The drawing under review shows one solid part. Ordinate dimensions are in mm from its lowest x, y, z. A direction names the side the tool comes from. Round coordinates to 2 decimals unless told otherwise and drop trailing zeros. Write each loop counter-clockwise with the first axis right and the second up, starting at its lowest first coordinate (ties: lowest second). Pieces come first, ordered by that corner, then holes. Notation, with made-up numbers: (58, 10) -> (95, 10) arc R17 cw to (95, 39) -> close; hole circle Ø11 at (84, 20.25). An arc over 180 degrees is marked (long way). Write item = value, one per line. Start each with the question number.
Item 1: Mouldability with a two-part tool opening along Z and no side actions: class the marked faces 4, 5, 6 and 7 as released by +Z, released by -Z, zero draft, split by the parting line, or undercut.
Item 2: Add section B-B, the plane z = 27.5. State the section outline as (x, y) points (1 decimal), then the cut area to 3 significant figures.
Item 3: Add section D-D, the plane z = 47. State the section outline as (x, y) points (1 decimal).
Item 4: Add section C-C, the plane y = 28. State the section outline as (x, z) points.
Item 5: Machinability: for the marked faces 1, 2 and 3, which of the approach directions +Z, -Z, +X, -X, +Y, -Y give a long, thin tool a straight path to every point of the face, cutting with its end or side? Answer none if there is none.
Item 6: To check wall thickness, follow L1, parallel to Y at x = 24.5, z = 45.5; L2, parallel to X at y = 8, z = 27 (1 decimal); L3, parallel to Z at x = 85, y = 6.75. State the ranges of each line that lie inside material, in increasing order.
Item 7: Add section A-A, the plane x = 17.5. State the section outline as (y, z) points.
Item 8: For pin 1 Ø2.5 at (y, z) = (1.5, 16) entering from -X (3 decimals); pin 2 Ø9 at (x, y) = (21.5, 40) entering from -Z; pin 3 Ø6 at (x, z) = (37.5, 41) entering from -Y, all flat-tipped, find the tip position at first contact; note any pin that passes through.
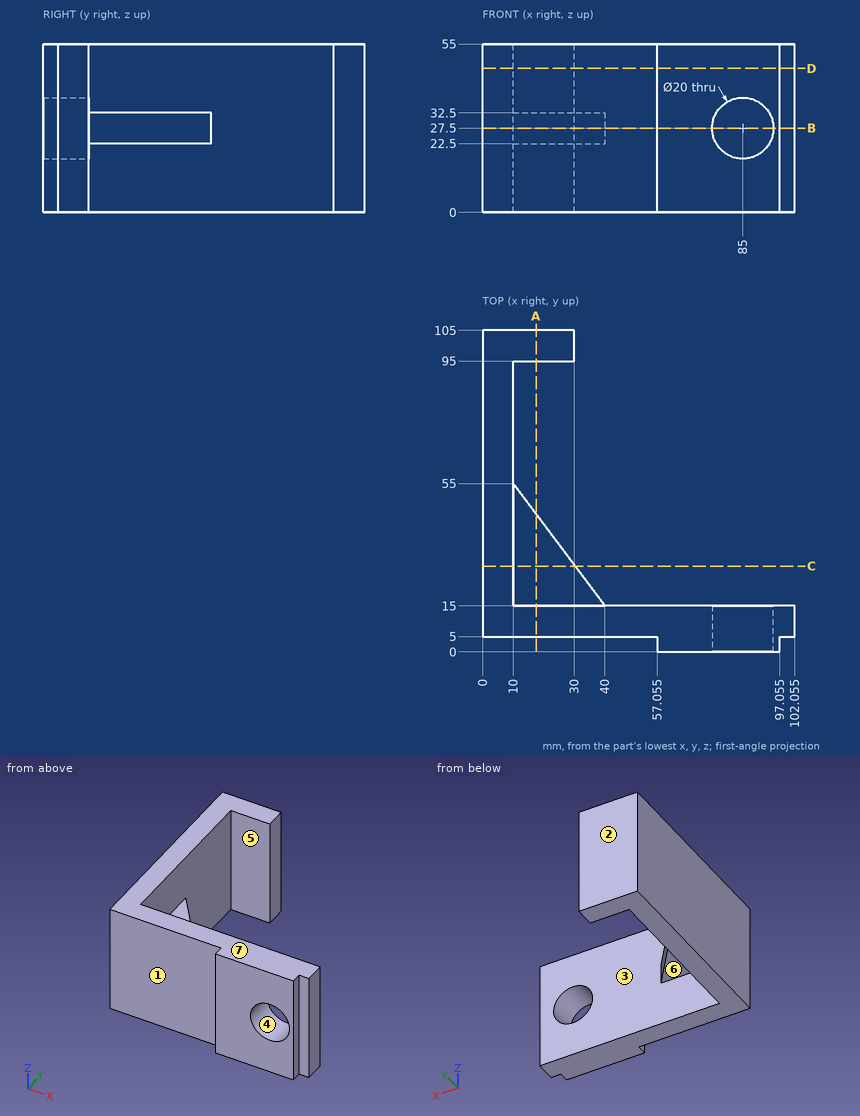
Result set:
q1.face_4 = undercut
q1.face_5 = zero draft
q1.face_6 = released by -Z
q1.face_7 = released by +Z
q2.outline = (0, 5) -> (57.1, 5) -> (57.1, 0) -> (75, 0) -> (75, 15) -> (40, 15) -> (10, 55) -> (10, 95) -> (30, 95) -> (30, 105) -> (0, 105) -> close; (95, 0) -> (97.1, 0) -> (97.1, 5) -> (102.1, 5) -> (102.1, 15) -> (95, 15) -> close
q2.area = 2,620 mm²
q3.outline = (0, 5) -> (57.1, 5) -> (57.1, 0) -> (97.1, 0) -> (97.1, 5) -> (102.1, 5) -> (102.1, 15) -> (10, 15) -> (10, 95) -> (30, 95) -> (30, 105) -> (0, 105) -> close
q4.outline = (0, 0) -> (10, 0) -> (10, 22.5) -> (30.25, 22.5) -> (30.25, 32.5) -> (10, 32.5) -> (10, 55) -> (0, 55) -> close
q5.face_1 = +Z, -Z, -X, -Y
q5.face_2 = +Z, -Z, +X, -X, +Y
q5.face_3 = +X
q6.L1 = 5 to 15, 95 to 105
q6.L2 = 0 to 75, 95 to 102.1
q6.L3 = 0 to 17.5, 37.5 to 55
q7.outline = (5, 0) -> (15, 0) -> (15, 22.5) -> (45, 22.5) -> (45, 32.5) -> (15, 32.5) -> (15, 55) -> (5, 55) -> close; (95, 0) -> (105, 0) -> (105, 55) -> (95, 55) -> close
q8.pin_1 = 57.055
q8.pin_2 = 22.5
q8.pin_3 = 5
